from build123d import *

# Parameters (mm, degrees)
SKETCH1_R           = 5
BOSS_EXTRUDE1_DEPTH = 126
CHAMFER1_SIZE       = 0.75
SKETCH2_W           = 1
SKETCH2_H           = 0.8


with BuildPart() as part:
    # Sketch1 → Boss-Extrude1 (new body)
    with BuildSketch(Plane(origin=(0, 0, 0), x_dir=(1, 0, 0), z_dir=(0, 1, 0))):
        with Locations(Location((0, 0, 0), (0, 0, 270))):
            Circle(SKETCH1_R)
    extrude(amount=BOSS_EXTRUDE1_DEPTH)

    # Chamfer1
    chamfer1_edges = [part.edges().sort_by_distance(p)[0] for p in [
        (0, 0, -5),
        (0, 126, -5),
    ]]
    chamfer(chamfer1_edges, length=CHAMFER1_SIZE)

    # Sketch2 → Cut-Revolve1 (revolve, cut)
    with BuildSketch(Plane.XY, mode=Mode.PRIVATE) as cut_revolve1_sk:
        with Locations((-4.5, 47.8)):
            Rectangle(SKETCH2_W, SKETCH2_H)
        with Locations((-4.5, 71.6)):
            Rectangle(SKETCH2_W, SKETCH2_H)
    revolve(cut_revolve1_sk.sketch.rotate(Axis((0, 111.50643277, 0), (0, -1, 0)), 270), axis=Axis((0, 111.50643277, 0), (0, -1, 0)), mode=Mode.SUBTRACT)


solid = part.part
Source: CAD feature listing. Evaluate the final solid. Frame: model axes, mm. A direction names the side the tool comes from. Round coordinates to 2 decimals unless told otherwise and drop trailing zeros. Loops run counter-clockwise (first coordinate to the right, second up) from the corner with the lowest first, then second, coordinate; pieces in that order, holes last.
Q1. Access query for faces 4 (the face through (-4.88, 59.54, -1.08)), 5 (the face through (3.905, 47.806, -0.867)). Directions: +Z, -Z, +X, -X, +Y, -Y. A direction counts if a zero-diameter tool reaches every point of the face in a straight line with its end or side. Return the directions, or none.
Q2. Section A-A, the plane y = 105. Return loops of the section in (x, z).
Q3. Mould query, pull axis Y, two halves, no side actions, for faces 1 (the face through (-4.88, 98.25, -1.08)), 2 (the face through (0, 0, 0)), 3 (the face through (3.905, 71.606, -0.867)). Classes: pulls with the +Y half, pulls with the -Y half, needs draft (parallel to the pull), parting line crosses it, or undercut.
Q4. Ray query, line 1 (Y direction, x = -2.75, z = 3.75); line 2 (X direction, y = 74, z = 0.25); line 3 (X direction, y = 81.5, z = -3). Return the intervals inside material, ascending.
Q5. First-contact query: P1, Ø1, axis at x = 2.5, y = 39.5, coming from the -Z side; P2, Ø4, axis at x = 2.5, y = 99.5, coming from the +Z side. Flat tips, straight axial feed; report the tip coordinate or a pass-through.
Solutions:
1. face 4: +Y, -Y
1. face 5: none
2. outline: circle Ø10 at (0, 0)
3. face 1: needs draft
3. face 2: pulls with the -Y half
3. face 3: undercut
4. line 1: y = 0.4 to 47.4, 48.2 to 71.2, 72 to 125.6
4. line 2: x = -4.99 to 4.99
4. line 3: x = -4 to 4
5. P1: stops at z = -4.58
5. P2: stops at z = 4.97
